from build123d import *

# Parameters (mm, degrees)
SKETCH1_W           = 90
SKETCH1_H           = 60
BOSS_EXTRUDE1_DEPTH = 50
SKETCH2_W           = 70
SKETCH2_H           = 50
CUT_EXTRUDE1_DEPTH  = 40
CUT_EXTRUDE3_START  = 50
SKETCH1_5_R         = 2.25
CUT_EXTRUDE3_DEPTH  = 40
CUT_EXTRUDE4_START  = 50
SKETCH1_6_R         = 15
SKETCH1_6_R_2       = 2.25
CUT_EXTRUDE4_DEPTH  = 3
SKETCH3_R           = 5
CUT_EXTRUDE5_DEPTH  = 91
CUT_EXTRUDE7_START  = -10
SKETCH3_3_R         = 11
SKETCH3_3_R_2       = 5
SKETCH3_3_R_3       = 1.6
CUT_EXTRUDE7_DEPTH  = 7
CUT_EXTRUDE8_START  = -80
SKETCH3_4_R         = 11
SKETCH3_4_R_2       = 5
SKETCH3_4_R_3       = 1.6
CUT_EXTRUDE8_DEPTH  = 7
SKETCH3_5_R         = 1.6
CUT_EXTRUDE9_DEPTH  = 91
SKETCH4_R           = 2.25
CUT_EXTRUDE10_DEPTH = 60


with BuildPart() as part:
    # Sketch1 → Boss-Extrude1 (new body)
    with BuildSketch(Plane(origin=(0, 0, 0), x_dir=(1, 0, 0), z_dir=(0, 1, 0))):
        Rectangle(SKETCH1_W, SKETCH1_H)
    extrude(amount=BOSS_EXTRUDE1_DEPTH)

    # Sketch2 → Cut-Extrude1 (cut)
    with BuildSketch(Plane.XZ):
        Rectangle(SKETCH2_W, SKETCH2_H)
    extrude(amount=-CUT_EXTRUDE1_DEPTH, mode=Mode.SUBTRACT)

    # Sketch1<5> → Cut-Extrude3 (cut)
    with BuildSketch(Plane(origin=(0, 0, 0), x_dir=(1, 0, 0), z_dir=(0, 1, 0)).offset(CUT_EXTRUDE3_START)):
        with Locations((0, -10)):
            Circle(SKETCH1_5_R)
        with Locations((-10, 0)):
            Circle(SKETCH1_5_R)
        with Locations((0, 10)):
            Circle(SKETCH1_5_R)
        with Locations((10, 0)):
            Circle(SKETCH1_5_R)
    extrude(amount=-CUT_EXTRUDE3_DEPTH, mode=Mode.SUBTRACT)

    # Sketch1<6> → Cut-Extrude4 (cut)
    with BuildSketch(Plane(origin=(0, 0, 0), x_dir=(1, 0, 0), z_dir=(0, 1, 0)).offset(CUT_EXTRUDE4_START)):
        Circle(SKETCH1_6_R)
        with Locations((-10, 0)):
            Circle(SKETCH1_6_R_2, mode=Mode.SUBTRACT)
        with Locations((0, -10)):
            Circle(SKETCH1_6_R_2, mode=Mode.SUBTRACT)
        with Locations((10, 0)):
            Circle(SKETCH1_6_R_2, mode=Mode.SUBTRACT)
        with Locations((0, 10)):
            Circle(SKETCH1_6_R_2, mode=Mode.SUBTRACT)
    extrude(amount=-CUT_EXTRUDE4_DEPTH, mode=Mode.SUBTRACT)

    # Sketch3 → Cut-Extrude5 (cut, through all)
    with BuildSketch(Plane.ZY.offset(45)):
        with Locations((0, 25)):
            Circle(SKETCH3_R)
    extrude(amount=-CUT_EXTRUDE5_DEPTH, mode=Mode.SUBTRACT)

    # Sketch3<3> → Cut-Extrude7 (cut)
    with BuildSketch(Plane.ZY.offset(45).offset(CUT_EXTRUDE7_START)):
        with Locations((0, 25)):
            Circle(SKETCH3_3_R)
        with Locations((0, 25)):
            Circle(SKETCH3_3_R_2, mode=Mode.SUBTRACT)
        with Locations((-12.02081528, 37.02081528)):
            Circle(SKETCH3_3_R_3)
        with Locations((12.02081528, 37.02081528)):
            Circle(SKETCH3_3_R_3)
        with Locations((12.02081528, 12.97918472)):
            Circle(SKETCH3_3_R_3)
        with Locations((-12.02081528, 12.97918472)):
            Circle(SKETCH3_3_R_3)
    extrude(amount=CUT_EXTRUDE7_DEPTH, mode=Mode.SUBTRACT)

    # Sketch3<4> → Cut-Extrude8 (cut)
    with BuildSketch(Plane.ZY.offset(45).offset(CUT_EXTRUDE8_START)):
        with Locations((0, 25)):
            Circle(SKETCH3_4_R)
        with Locations((0, 25)):
            Circle(SKETCH3_4_R_2, mode=Mode.SUBTRACT)
        with Locations((-12.02081528, 37.02081528)):
            Circle(SKETCH3_4_R_3)
        with Locations((12.02081528, 37.02081528)):
            Circle(SKETCH3_4_R_3)
        with Locations((12.02081528, 12.97918472)):
            Circle(SKETCH3_4_R_3)
        with Locations((-12.02081528, 12.97918472)):
            Circle(SKETCH3_4_R_3)
    extrude(amount=-CUT_EXTRUDE8_DEPTH, mode=Mode.SUBTRACT)

    # Sketch3<5> → Cut-Extrude9 (cut, through all)
    with BuildSketch(Plane.ZY.offset(45)):
        with Locations((-12.02081528, 37.02081528)):
            Circle(SKETCH3_5_R)
        with Locations((12.02081528, 37.02081528)):
            Circle(SKETCH3_5_R)
        with Locations((12.02081528, 12.97918472)):
            Circle(SKETCH3_5_R)
        with Locations((-12.02081528, 12.97918472)):
            Circle(SKETCH3_5_R)
    extrude(amount=-CUT_EXTRUDE9_DEPTH, mode=Mode.SUBTRACT)

    # Sketch4 → Cut-Extrude10 (cut)
    with BuildSketch(Plane.XY.offset(30)):
        with Locations((-31.833799112, 5)):
            Circle(SKETCH4_R)
        with Locations((-31.833799112, 45.010389169)):
            Circle(SKETCH4_R)
        with Locations((13.166200888, 5)):
            Circle(SKETCH4_R)
        with Locations((13.166200888, 45.10389169)):
            Circle(SKETCH4_R)
    extrude(amount=-CUT_EXTRUDE10_DEPTH, mode=Mode.SUBTRACT)


solid = part.part
The model under review builds one solid part; all positions refer to its coordinate system, in mm. A direction names the side the tool comes from. Round coordinates to 2 decimals unless told otherwise and drop trailing zeros. Loops run counter-clockwise (first coordinate to the right, second up) from the corner with the lowest first, then second, coordinate; pieces in that order, holes last. Notation, with made-up numbers: M -1,81.25 L 26,81.25 A16 ccw 26,94.25 Z; hole C 66.5,-17.5 d9. An arc over 180 degrees is marked long. Answer as CSV lines item,"result". Start each with the question number.
Item 1: Mouldability with a two-part tool opening along Z and no side actions: class faces 1 (the face through (12.87, 7.23, 27.54)), 2 (the face through (-1, 25, 30)), 3 (the face through (43.48, 20.12, -1.08)) as released by +Z, released by -Z, zero draft, split by the parting line, or undercut.
Item 2: Insertion check: P1, Ø5, axis at x = 0, z = 10, coming from the +Y side; P2, Ø17.5, axis at y = 24.5, z = 3.5, coming from the +X side; P3, Ø3.5, axis at x = 13.17, y = 5, coming from the +Z side; P4, Ø10, axis at x = 19, z = -14.5, coming from the -Y side. Each pin has a flat end and moves straight along its axis. Give the tip position at first contact, or say it passes through.
Item 3: For faces 4 (the face through (-1, 0, 26)), 5 (the face through (0, 20, -25)), 6 (the face through (9, 50, -14)), 7 (the face through (42, 20, 2)), 8 (the face through (-2, 47, 0)), list the 3-axis set-ups (+Z, -Z, +X, -X, +Y, -Y) from which the entire face can be reached by the end or side of a thin tool; tool diameter is ignored.
Item 4: Consider section A-A (x = 0). Write out the cut boundary in (y, z), then the cut area to 3 significant figures.
Item 5: Consider section B-B (y = 25). Write out the cut boundary in (x, z).
Item 6: Wall thickness on line 1 (Z direction, x = 0, y = 42.25); line 2 (Z direction, x = 0, y = 10); line 3 (X direction, y = 7, z = -1): over which ranges is each line inside the solid? List them lowest first. Write a range as [from, to].
Item 7: Consider section D-D (x = -10). Write out the cut boundary in (y, z), then the cut area to 3 significant figures.
Item 8: Consider section C-C (y = 5). Write out the cut boundary in (x, z).
Answer:
1,face 1,"zero draft"
1,face 2,"released by +Z"
1,face 3,"undercut"
2,P1,"stops at y = 47"
2,P2,"stops at x = 45"
2,P3,"passes through"
2,P4,"stops at y = 40"
3,face 4,"+Z, -Z, +X, -X, -Y"
3,face 5,"-Y"
3,face 6,"+Z, -Z, +X, -X, +Y"
3,face 7,"none"
3,face 8,"+Y"
4,outline,"M 0,-30 L 50,-30 L 50,-15 L 47,-15 L 47,-12.25 L 40,-12.25 L 40,-25 L 0,-25 Z; M 0,25 L 40,25 L 40,12.25 L 47,12.25 L 47,15 L 50,15 L 50,30 L 0,30 Z; M 40,-7.75 L 47,-7.75 L 47,7.75 L 40,7.75 Z"
4,area,"847 mm^2"
5,outline,"M -45,-30 L 45,-30 L 45,-5 L 42,-5 L 42,-11 L 35,-11 L 35,-25 L -35,-25 L -35,-11 L -42,-11 L -42,-5 L -45,-5 Z; M -45,5 L -42,5 L -42,11 L -35,11 L -35,25 L 35,25 L 35,11 L 42,11 L 42,5 L 45,5 L 45,30 L -45,30 Z"
6,line 1,"z = [-30, -12.25], [-7.75, 7.75], [12.25, 30]"
6,line 2,"z = [-30, -25], [25, 30]"
6,line 3,"x = [-45, -35], [35, 45]"
7,outline,"M 0,-30 L 50,-30 L 50,-11.18 L 47,-11.18 L 47,-2.25 L 40,-2.25 L 40,-25 L 0,-25 Z; M 0,25 L 40,25 L 40,2.25 L 47,2.25 L 47,11.18 L 50,11.18 L 50,30 L 0,30 Z"
7,area,"901 mm^2"
8,outline,"M -45,-30 L -34.08,-30 L -34.08,-25 L -35,-25 L -35,25 L -34.08,25 L -34.08,30 L -45,30 Z; M -29.58,-30 L 10.92,-30 L 10.92,-25 L -29.58,-25 Z; M -29.58,25 L 10.92,25 L 10.92,30 L -29.58,30 Z; M 15.42,-30 L 45,-30 L 45,30 L 15.42,30 L 15.42,25 L 35,25 L 35,-25 L 15.42,-25 Z"
